Check sheet for the modelled part. Datum: model origin and axes. Units: mm. A direction names the side the tool comes from. Round coordinates to 2 decimals unless told otherwise and drop trailing zeros. Order: outer loops, then holes, each group sorted by start corner. A loop starts at its lowest first (then second) coordinate and runs counter-clockwise, first axis right, second up.
```python
from build123d import *

# Parameters (mm, degrees)
F0_W     = 126.238
F0_H     = 156.718
F1_DEPTH = 25.4
F3_DEPTH = 124.46
F4_DEPTH = 152.4
F5_W     = 7.62
F5_H     = 139.9129815726
F6_DEPTH = 7.62
F8_DEPTH = 152.4


with BuildPart() as f1:
    # F0 (on Front) → F1 (new body)
    with BuildSketch(Plane.XZ):
        with Locations((-22.7268721203, 17.8661712823)):
            Rectangle(F0_W, F0_H)
    extrude(amount=F1_DEPTH)

    # F2 (on face) → F3 (cut)
    with BuildSketch(Plane(origin=(-85.8458721203, 0, 0), x_dir=(0, -1, 0), z_dir=(-1, 0, 0))):
        Polygon((4.9062082183, -55.539762938), (0, 84.2871712823), (0, -60.4928287177), (4.9062082183, -60.4928287177), align=None)
    extrude(amount=-F3_DEPTH, mode=Mode.SUBTRACT)

    # F2 (on face) → F4 (cut)
    with BuildSketch(Plane(origin=(-85.8458721203, 0, 0), x_dir=(0, -1, 0), z_dir=(-1, 0, 0))):
        Polygon((0, 84.2871712823), (2.54, 84.2871712823), (7.4462082183, -55.539762938), (7.4462082183, -60.4928287177), (25.4, -60.4928287177), (25.4, 96.2251712823), (0, 96.2251712823), align=None)
    extrude(amount=-F4_DEPTH, mode=Mode.SUBTRACT)

    # F5 (on face) → F6 (join)
    with BuildSketch(Plane(origin=(0, -5.4906847606, 0.1926556056), x_dir=(1, 0, 0), z_dir=(0, -0.9993849938, 0.0350661401))):
        with Locations((-82.0358721203, 14.1897753664)):
            Rectangle(F5_W, F5_H)
    extrude(amount=F6_DEPTH)

    # F7 (on face) → F8 (cut)
    with BuildSketch(Plane(origin=(0, 2.9506847606, 84.0945156767), x_dir=(1, 0, 0), z_dir=(0, 0.0350661401, 0.9993849938))):
        with BuildLine():
            Line((-78.2258721203, -13.1140636438), (-78.2258721203, -5.4940636438))
            ThreePointArc((-78.2258721203, -5.4940636438), (-83.6140257929, -7.7259099712), (-85.8458721203, -13.1140636438))
            Line((-85.8458721203, -13.1140636438), (-78.2258721203, -13.1140636438))
        make_face()
    extrude(amount=-F8_DEPTH, mode=Mode.SUBTRACT)


solid = f1.part
```
Item 1: Go/stop test with flat-tipped pins: P1, Ø5, axis at x = -60.5, z = -3.5, coming from the -Y side; P2, Ø2.5, axis at x = -3.5, z = -58, coming from the -Y side; P3, Ø1.3, axis at x = 2, y = -1, coming from the +Z side. Record where each tip stops, or that it passes through.
Answer:
P1: stops at y = -5.71
P2: stops at y = -7.45
P3: stops at z = 84.29
Item 2: Access from +Z, -Z, +X, -X, +Y, -Y to the whole of each face (thin tool, end or side, straight path). Record for faces 4 (the flat face through (-23, -6, -60.493)), 5 (the flat face through (38.614, -2, -3)).
Answer:
face 4: -Z, +X, -X, +Y, -Y
face 5: -Z, -X, +Y
Item 3: Sectioned sample at A-A (x = 28.5). Record the cut outline in (y, z).
Answer:
outline: (-7.45, -60.49) - (-4.91, -60.49) - (-4.91, -55.54) - (0, 84.29) - (-2.54, 84.29) - (-7.45, -55.54) - close
Item 4: Scan lines: line 1 along X through (y, z) = (-11.75, -14); line 2 along Y through (x, z) = (-60, -33); line 3 along Y through (x, z) = (-66.5, 20). Record each from-to range of solid material in increasing order.
Answer:
line 1: x = -85.85 to -85.61
line 2: y = -6.66 to -4.12
line 3: y = -4.8 to -2.26
Item 5: Release check for a two-part mould opening along X. For faces 1 (the flat face through (-85.846, -7, 11)), 2 (the flat face through (-24, -4.906, -58)), 3 (the cylindrical face through (-83.554, -7.13, 15.429)) record: released by +X, released by -X, zero draft, split by the parting line, or undercut.
Answer:
face 1: released by -X
face 2: zero draft
face 3: released by +X
